Here's the drawing with two shaded views (mm, measured from the low corner). I have some questions. A direction names the side the tool comes from. Coordinates: 2 decimals unless noted, no trailing zeros. Write each loop counter-clockwise with the first axis right and the second up, starting at its lowest first coordinate (ties: lowest second). Pieces come first, ordered by that corner, then holes.
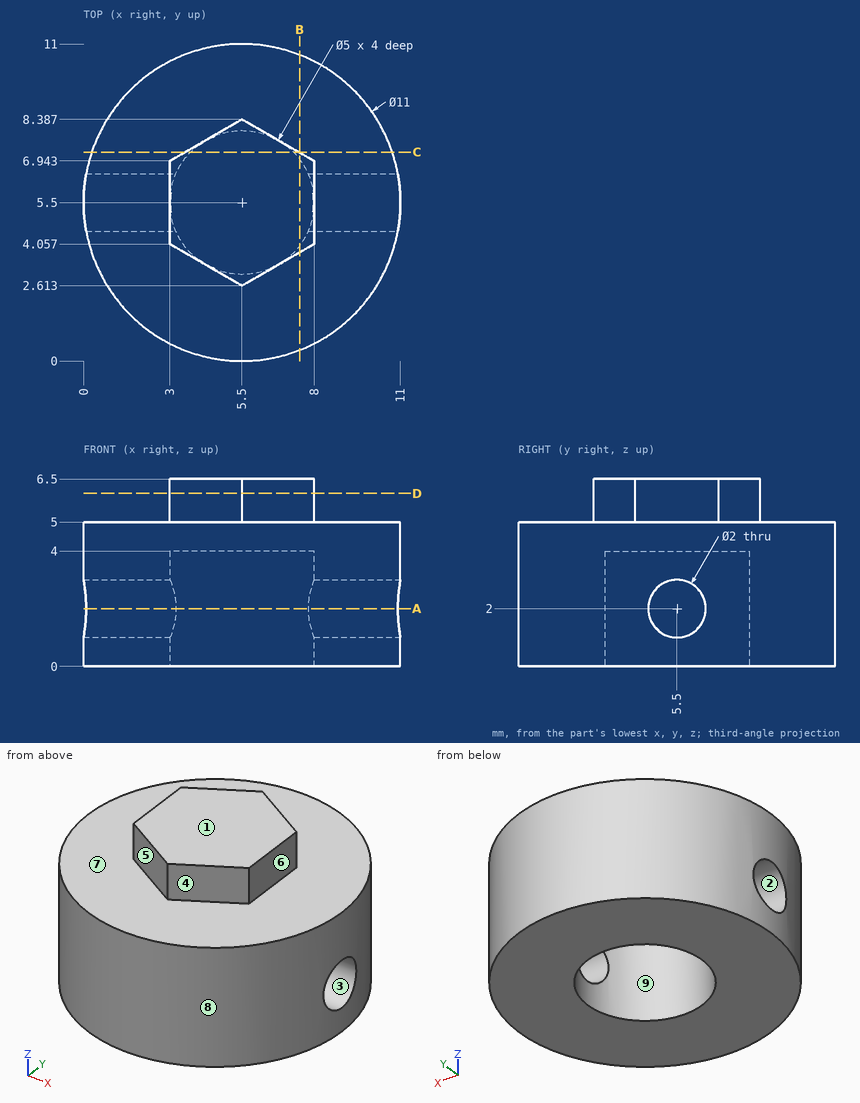
1. If we section it at A-A, the plane z = 2: List the corners of the cut face in (x, y) for me.
2. We'd pull the mould along Y, two halves only. Please class the marked faces 1, 2, 3 and 4: released by +Y, released by -Y, zero draft, split by the parting line, or undercut.
3. If we section it at B-B, the plane x = 7.5: List the corners of the cut face in (y, z) for me.
4. If I drill on L1, parallel to Y at x = 5.5, z = 1.35; L2, parallel to X at y = 6.75, z = 5.25; L3, parallel to Z at x = 3.5, y = 2.75, over which ranges is the centre line in solid material (lowest first)?
5. If we section it at D-D, the plane z = 6: List the corners of the cut face in (x, y) for me.
6. If we section it at C-C, the plane y = 7.25: List the corners of the cut face in (x, z) for me (1 decimal).
7. I'm going to push flat-ended pins straight in: P1, Ø1.2, axis at y = 5, z = 5.5, coming from the +X side; P2, Ø1.8, axis at y = 5.5, z = 2, coming from the +X side; P3, Ø4, axis at x = 5.5, y = 5.5, coming from the -Z side; P4, Ø2, axis at y = 3.5, z = 2, coming from the -X side. Where does each tip first touch, or does it pass through?
8. Which directions (+Z, -Z, +X, -X, +Y, -Y) give clear straight access to the entire face, cutting with the end or side of a thin tool? Please do the marked faces 5, 6, 7, 8 and 9.
Answers:
1. outline: (0.09, 4.5) arc R5.5 ccw to (10.91, 4.5) - (7.79, 4.5) arc R2.5 cw to (3.21, 4.5) - close; (0.09, 6.5) - (3.21, 6.5) arc R2.5 cw to (7.79, 6.5) - (10.91, 6.5) arc R5.5 ccw to start
2. face 1: zero draft
2. face 2: undercut
2. face 3: undercut
2. face 4: released by -Y
3. outline: (0.38, 0) - (4, 0) - (4, 4) - (7, 4) - (7, 0) - (10.62, 0) - (10.62, 5) - (7.23, 5) - (7.23, 6.5) - (3.77, 6.5) - (3.77, 5) - (0.38, 5) - close
4. L1: y = 0 to 3, 8 to 11
4. L2: x = 3 to 8
4. L3: z = 0 to 5
5. outline: (3, 4.06) - (5.5, 2.61) - (8, 4.06) - (8, 6.94) - (5.5, 8.39) - (3, 6.94) - close
6. outline: (0.3, 0) - (3.7, 0) - (3.7, 4) - (7.3, 4) - (7.3, 0) - (10.7, 0) - (10.7, 5) - (7.5, 5) - (7.5, 6.5) - (3.5, 6.5) - (3.5, 5) - (0.3, 5) - close
7. P1: stops at x = 11
7. P2: passes through
7. P3: stops at z = 4
7. P4: stops at x = 0.09
8. face 5: +Z, -X, -Y
8. face 6: +Z, +X, +Y, -Y
8. face 7: +Z
8. face 8: +Z, -Z
8. face 9: -Z
